```python
from build123d import *

# Parameters (mm, degrees)
SKETCH2_R           = 4
SKETCH2_R_2         = 1.35255
BOSS_EXTRUDE1_DEPTH = 2.032
SKETCH5_R           = 1.5875
SKETCH5_R_2         = 1.35255
CUT_EXTRUDE1_DEPTH  = 3.032


with BuildPart() as part:
    # Sketch2 → Boss-Extrude1 (new body)
    with BuildSketch(Plane.XY):
        with BuildLine():
            Line((64.594184148, -5.687884281), (43.406299867, 15.5))
            Line((43.406299867, 15.5), (0, 15.5))
            Line((0, 15.5), (-6.633092705, 11.758064516))
            ThreePointArc((-6.633092705, 11.758064516), (-13.306426587, -2.277940187), (-2.344250399, -13.294904666))
            Line((-2.344250399, -13.294904666), (15.832748501, -16.5))
            Line((15.832748501, -16.5), (53.78206843, -16.5))
            Line((53.78206843, -16.5), (64.594184148, -5.687884281))
        make_face()
        Circle(SKETCH2_R, mode=Mode.SUBTRACT)
        with Locations((24.053244616, 11.867587507)):
            Circle(SKETCH2_R_2, mode=Mode.SUBTRACT)
    extrude(amount=BOSS_EXTRUDE1_DEPTH)

    # Sketch5 → Cut-Extrude1 (cut, through all)
    with BuildSketch(Plane(origin=(0, 0, 0), x_dir=(-1, 0, 0), z_dir=(0, 0, -1))):
        with Locations((-41.514925917, -0.030322925)):
            Circle(SKETCH5_R)
        with Locations((-52.291233263, -10.80663027)):
            Circle(SKETCH5_R)
        with Locations((-45.107028366, 3.561779523)):
            Circle(SKETCH5_R_2)
        with Locations((-55.883335711, -7.214527822)):
            Circle(SKETCH5_R_2)
    extrude(amount=-CUT_EXTRUDE1_DEPTH, mode=Mode.SUBTRACT)


solid = part.part
```
Source: CAD feature listing. Evaluate the final solid. Frame: model axes, mm. Coordinates: 2 decimals unless noted, no trailing zeros. Write each loop counter-clockwise with the first axis right and the second up, starting at its lowest first coordinate (ties: lowest second). Pieces come first, ordered by that corner, then holes. Notation, with made-up numbers: (-22, 68.25) -> (-7, 68.25) arc R16 cw to (-7, 87.25) -> close; hole circle Ø6 at (64.25, -8). An arc over 180 degrees is marked (long way). Return JSON: item names as keys, results as strings. Group by question number.
1) Contact query for flat-ended pins moving along their axis: P1, Ø2, axis at x = 55.88, y = -7.21, coming from the -Z side; P2, Ø1.5, axis at x = 36, y = 8, coming from the -Z side. Output: stop coordinate, or through.
2) Ray query, line 1 along X through (y, z) = (-0.5, 1.3); line 2 along Y through (x, z) = (24, 0.2); line 3 along X through (y, z) = (-1, 0.2). Return the intervals inside material, ascending.
3) Mould query, pull axis Y, two halves, no side actions, for faces 1 (the face through (25, 0, 0)), 2 (the face through (46.46, 3.62, 1)), 3 (the face through (35, -16.5, 1)). Classes: +Y half, -Y half, draft (parallel to the pull), parting line (faces both ways), or undercut.
4) Section query D-D, the plane y = -14. Return loops of the section in (x, z), plus the area to 3 significant figures.
5) Section query B-B, the plane x = 53. Return loops of the section in (y, z).
6) Section query C-C, the plane z = 1.6. Return loops of the section in (x, y) (1 decimal).
7) Section query A-A, the plane y = -2.5. Return loops of the section in (x, z), plus the area to 3 significant figures.
From the geometry:
{
 "1": {"P1": "through", "P2": "z = 0"},
 "2": {"line 1": "-13.49 to -3.97, 3.97 to 40, 43.03 to 59.41", "line 2": "-16.5 to 10.52, 13.22 to 15.5", "line 3": "-13.46 to -3.87, 3.87 to 40.26, 42.77 to 59.91"},
 "3": {"face 1": "draft", "face 2": "undercut", "face 3": "-Y half"},
 "4": {"outline": "(1.65, 0) -> (56.28, 0) -> (56.28, 2.03) -> (1.65, 2.03) -> close", "area": "111 mm²"},
 "5": {"outline": "(-16.5, 0) -> (-12.23, 0) -> (-12.23, 2.03) -> (-16.5, 2.03) -> close; (-9.39, 0) -> (5.91, 0) -> (5.91, 2.03) -> (-9.39, 2.03) -> close"},
 "6": {"outline": "(-6.6, 11.8) arc R13.5 ccw to (-2.3, -13.3) -> (15.8, -16.5) -> (53.8, -16.5) -> (64.6, -5.7) -> (43.4, 15.5) -> (0, 15.5) -> close; hole circle Ø8 at (0, 0); hole circle Ø2.7 at (24.1, 11.9); hole circle Ø3.2 at (41.5, 0); hole circle Ø2.7 at (45.1, 3.6); hole circle Ø3.2 at (52.3, -10.8); hole circle Ø2.7 at (55.9, -7.2)"},
 "7": {"outline": "(-13.27, 0) -> (-3.12, 0) -> (-3.12, 2.03) -> (-13.27, 2.03) -> close; (3.12, 0) -> (61.41, 0) -> (61.41, 2.03) -> (3.12, 2.03) -> close", "area": "139 mm²"}
}
